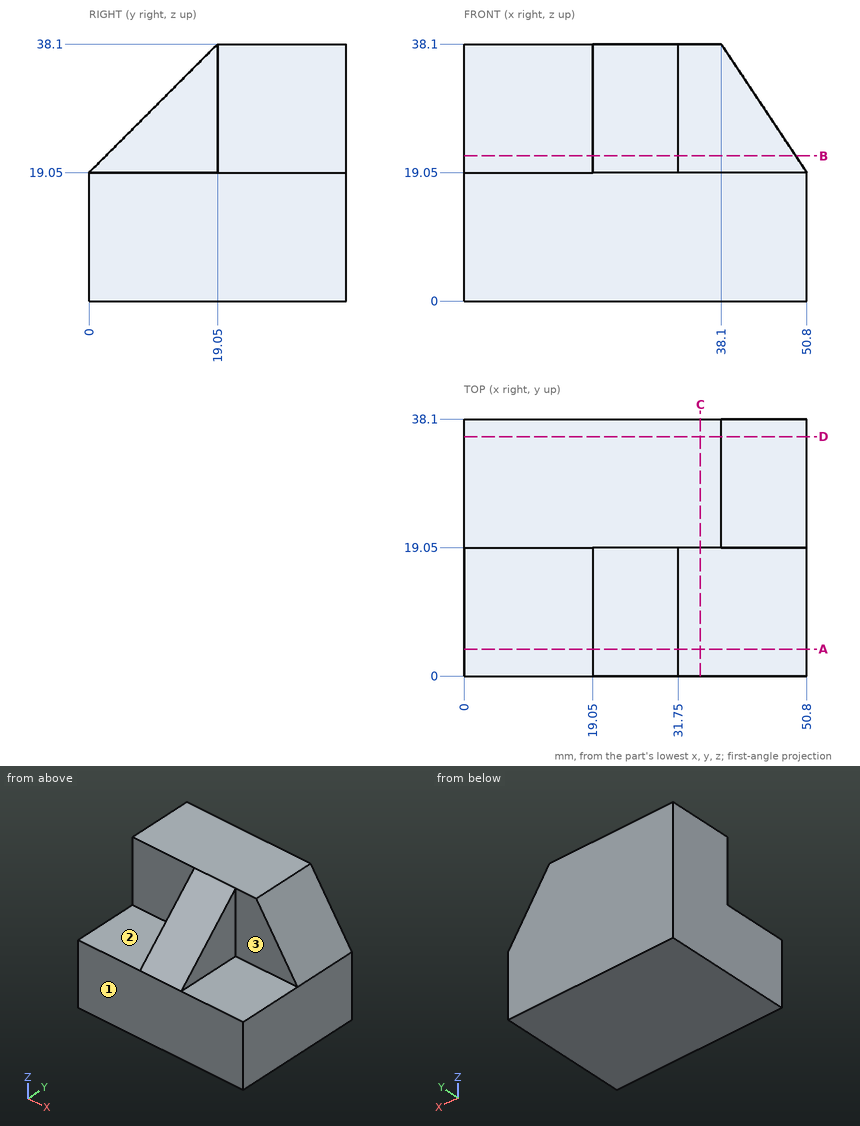
Verification items for this drawing (mm, ordinates from the low corner). A direction names the side the tool comes from. Give positions to 0.01 mm unless a question says otherwise; leave off trailing zeros. Loops run counter-clockwise (first coordinate to the right, second up) from the corner with the lowest first, then second, coordinate; pieces in that order, holes last. Notation, with made-up numbers: M 14,25 L 50,25 A19 cw 50,30 Z; hole C 58.5,-31.5 d8. An arc over 180 degrees is marked long. Answer as a JSON object with one key per item and string values. Group by question number.
Q1. Cross-section at B-B on z = 21.5. Record the cut outline in (x, y).
Q2. Go/stop test with flat-tipped pins: P1, Ø8, axis at y = 13, z = 7.5, coming from the -X side; P2, Ø5.5, axis at x = 45.5, y = 6.5, coming from the +Z side; P3, Ø9.5, axis at y = 13, z = 33, coming from the -X side; P4, Ø9.5, axis at x = 14, z = 27.5, coming from the -Y side. Record where each tip stops, or that it passes through.
Q3. Cross-section at A-A on y = 4. Record the cut outline in (x, z).
Q4. Access from +Z, -Z, +X, -X, +Y, -Y to the whole of each face (thin tool, end or side, straight path). Record for the marked faces 1, 2 and 3.
Q5. Cross-section at D-D on y = 35.5. Record the cut outline in (x, z).
Q6. Material ranges on line 1 along Y through (x, z) = (3, 31); line 2 along Z through (x, y) = (18.5, 9); line 3 along X through (y, z) = (8, 21), recorded low to high. Write a range as [from, to].
Q7. Cross-section at C-C on x = 35. Record the cut outline in (y, z).
Evaluation:
{
 "1": {"outline": "M 0,19.05 L 19.05,19.05 L 19.05,2.45 L 31.75,2.45 L 31.75,19.05 L 49.17,19.05 L 49.17,38.1 L 0,38.1 Z"},
 "2": {"P1": "stops at x = 0", "P2": "stops at z = 19.05", "P3": "stops at x = 19.05", "P4": "stops at y = 19.05"},
 "3": {"outline": "M 0,0 L 50.8,0 L 50.8,19.05 L 31.75,19.05 L 31.75,23.05 L 19.05,23.05 L 19.05,19.05 L 0,19.05 Z"},
 "4": {"face 1": "+Z, -Z, +X, -X, -Y", "face 2": "+Z, -X, -Y", "face 3": "+Z, +X, -Y"},
 "5": {"outline": "M 0,0 L 50.8,0 L 50.8,19.05 L 38.1,38.1 L 0,38.1 Z"},
 "6": {"line 1": "y = [19.05, 38.1]", "line 2": "z = [0, 19.05]", "line 3": "x = [19.05, 31.75]"},
 "7": {"outline": "M 0,0 L 38.1,0 L 38.1,38.1 L 19.05,38.1 L 19.05,19.05 L 0,19.05 Z"}
}
